```python
from build123d import *

# Parameters (mm, degrees)
F0_W     = 355.6
F0_H     = 254
F1_DEPTH = 190.5
F2_T     = -25.4
F4_D     = 5.08


with BuildPart() as f1:
    # F0 (on Top) → F1 (new body)
    with BuildSketch(Plane.XY):
        Rectangle(F0_W, F0_H)
    extrude(amount=F1_DEPTH)

    # F2
    f2_openings = [f1.faces().sort_by_distance(p)[0] for p in [
        (0, 0, 190.5),
    ]]
    offset(amount=F2_T, openings=f2_openings)

    # F4 (through all)
    with Locations(Plane.XY.offset(25.4)):
        with Locations((-127, 76.2), (-127, -76.2), (127, -76.2), (127, 76.2)):
            Hole(F4_D / 2)


solid = f1.part
```
Geometry: final body of the model. Coordinates: model frame, mm. A direction names the side the tool comes from. Give positions to 0.01 mm unless a question says otherwise; leave off trailing zeros. Loops run counter-clockwise (first coordinate to the right, second up) from the corner with the lowest first, then second, coordinate; pieces in that order, holes last. Notation, with made-up numbers: (-21.5, 32) -> (28.5, 32) arc R17 cw to (28.5, 61) -> close; hole circle Ø5 at (86.5, 61). An arc over 180 degrees is marked (long way). Use one line per item in the form item = value.
Item 1: Section query B-B on y = 13. Output: boundary loops of the cut face in (x, z), and give its area (3 significant figures).
A:
outline = (-177.8, 0) -> (177.8, 0) -> (177.8, 190.5) -> (152.4, 190.5) -> (152.4, 25.4) -> (-152.4, 25.4) -> (-152.4, 190.5) -> (-177.8, 190.5) -> close
area = 17,400 mm^2
Item 2: Draft query along X for faces 1 (the face through (152.4, -1, 107)), 2 (the face through (-177.8, -2, 94)), 3 (the face through (-2, -127, 94)). Return one class per face: pulls with the +X half, pulls with the -X half, needs draft (parallel to the pull), parting line crosses it, or undercut.
A:
face_1 = undercut
face_2 = pulls with the -X half
face_3 = needs draft
Item 3: Line query: probe 1 along X at (y, z) = (76.5, 17.5); probe 2 along Y at (x, z) = (-127, 17.25); probe 3 along Y at (x, z) = (99.5, 84). Output: solid intervals per line, ascending.
A:
probe_1 = -177.8 to -129.52, -124.48 to 124.48, 129.52 to 177.8
probe_2 = -127 to -78.74, -73.66 to 73.66, 78.74 to 127
probe_3 = -127 to -101.6, 101.6 to 127
Item 4: Section query A-A on z = 172.5. Output: boundary loops of the cut face in (x, y), and give its area (3 significant figures).
A:
outline = (-177.8, -127) -> (177.8, -127) -> (177.8, 127) -> (-177.8, 127) -> close; hole (-152.4, -101.6) -> (152.4, -101.6) -> (152.4, 101.6) -> (-152.4, 101.6) -> close
area = 28,400 mm^2
Item 5: Section query C-C on x = 21. Output: boundary loops of the cut face in (y, z), and give its area (3 significant figures).
A:
outline = (-127, 0) -> (127, 0) -> (127, 190.5) -> (101.6, 190.5) -> (101.6, 25.4) -> (-101.6, 25.4) -> (-101.6, 190.5) -> (-127, 190.5) -> close
area = 14,800 mm^2
Item 6: Access query for faces 4 (the face through (-2, -101.6, 107)), 5 (the face through (-2, 127, 94)). Directions: +Z, -Z, +X, -X, +Y, -Y. A direction counts if a zero-diameter tool reaches every point of the face in a straight line with its end or side. Return the directions, or none.
A:
face_4 = +Z
face_5 = +Z, -Z, +X, -X, +Y
Item 7: Pin query (flat end, axial travel): P1, Ø1, axis at x = -117.5, y = -32, coming from the +Z side. Return the tip coordinate at first contact, or that it passes through.
A:
P1 = 25.4
